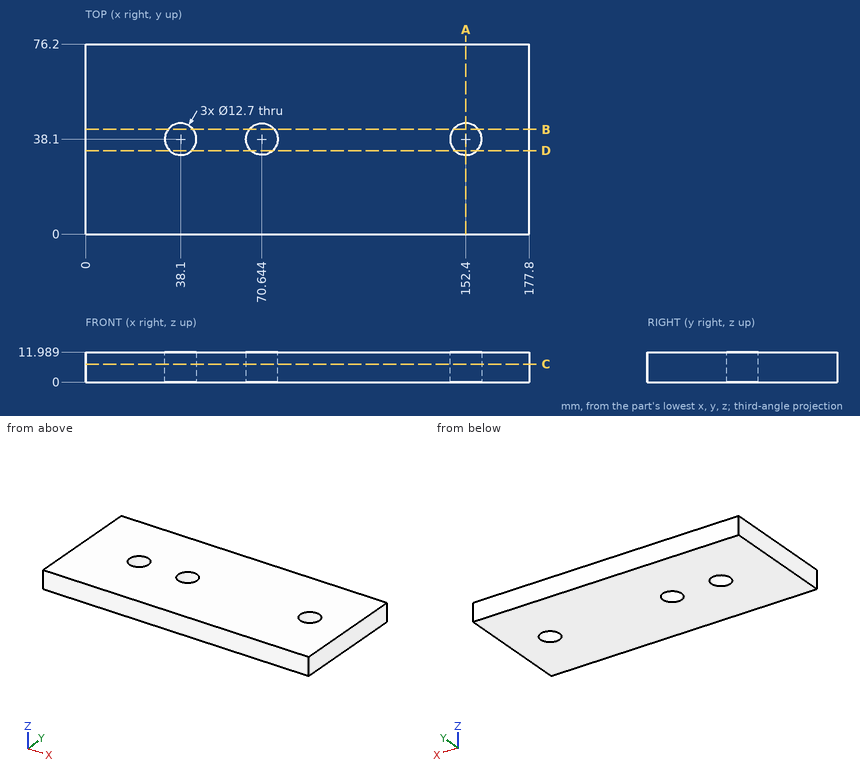
Design review of the part shown in the three views and the two pictorial views. Dimensions are in mm from the part's minimum x, y and z. Give positions to 0.01 mm unless a question says otherwise; leave off trailing zeros. Write each loop counter-clockwise with the first axis right and the second up, starting at its lowest first coordinate (ties: lowest second). Pieces come first, ordered by that corner, then holes. Notation, with made-up numbers: (9, 18.25) -> (17, 18.25) arc R9 cw to (17, 29.25) -> close; hole circle Ø6 at (87.5, 69.25). An arc over 180 degrees is marked (long way). Answer in a Markdown table with one row per item.
1) Add section C-C on z = 7.25. State the section outline as (x, y) points.
Worked answers:
| item | result |
|---|---|
| outline | (0, 0) -> (177.8, 0) -> (177.8, 76.2) -> (0, 76.2) -> close; hole circle Ø12.7 at (38.1, 38.1); hole circle Ø12.7 at (70.64, 38.1); hole circle Ø12.7 at (152.4, 38.1) |
2) Add section B-B on y = 42. State the section outline as (x, z) points (1 decimal), plus the area to 3 significant figures.
Worked answers:
| item | result |
|---|---|
| outline | (0, 0) -> (33.1, 0) -> (33.1, 12) -> (0, 12) -> close; (43.1, 0) -> (65.6, 0) -> (65.6, 12) -> (43.1, 12) -> close; (75.7, 0) -> (147.4, 0) -> (147.4, 12) -> (75.7, 12) -> close; (157.4, 0) -> (177.8, 0) -> (177.8, 12) -> (157.4, 12) -> close |
| area | 1,770 mm² |
3) Add section A-A on x = 152.4. State the section outline as (y, z) points.
Worked answers:
| item | result |
|---|---|
| outline | (0, 0) -> (31.75, 0) -> (31.75, 11.99) -> (0, 11.99) -> close; (44.45, 0) -> (76.2, 0) -> (76.2, 11.99) -> (44.45, 11.99) -> close |
4) Add section D-D on y = 33.5. State the section outline as (x, z) points.
Worked answers:
| item | result |
|---|---|
| outline | (0, 0) -> (33.72, 0) -> (33.72, 11.99) -> (0, 11.99) -> close; (42.48, 0) -> (66.27, 0) -> (66.27, 11.99) -> (42.48, 11.99) -> close; (75.02, 0) -> (148.02, 0) -> (148.02, 11.99) -> (75.02, 11.99) -> close; (156.78, 0) -> (177.8, 0) -> (177.8, 11.99) -> (156.78, 11.99) -> close |
5) For L1, parallel to X at y = 38, z = 6.5 (1 decimal); L2, parallel to Y at x = 152.4, z = 2.75; L3, parallel to Y at x = 157.5, z = 10.75 (1 decimal), list the stretches that pass through material, from the lowest coordinate up. Write a range as [from, to].
Worked answers:
| item | result |
|---|---|
| L1 | [0, 31.8], [44.4, 64.3], [77, 146.1], [158.7, 177.8] |
| L2 | [0, 31.75], [44.45, 76.2] |
| L3 | [0, 34.3], [41.9, 76.2] |
6) Clearance check with flat-ended pins moving along their axes: P1, Ø11.5, axis at x = 152.4, y = 38.1, coming from the +Z side; P2, Ø3, axis at x = 99.5, y = 67, coming from the -Z side. State where each tip first meets the part, or that it passes through.
Worked answers:
| item | result |
|---|---|
| P1 | through |
| P2 | z = 0 |
